from build123d import *

# Parameters (mm, degrees)
ESQUISSE1_R        = 46
BOSS_EXTRU_1_DEPTH = 41
ESQUISSE2_R        = 10
BOSS_EXTRU_2_DEPTH = 1.5
ESQUISSE3_R        = 8
BOSS_EXTRU_3_DEPTH = 3
ESQUISSE4_R        = 0.995
BOSS_EXTRU_4_DEPTH = 3


with BuildPart() as part:
    # Esquisse1 → Boss.-Extru.1 (new body)
    with BuildSketch(Plane(origin=(0, 0, 0), x_dir=(1, 0, 0), z_dir=(0, 1, 0))):
        with Locations(Location((0, 0, 0), (0, 0, 270))):
            Circle(ESQUISSE1_R)
    extrude(amount=BOSS_EXTRU_1_DEPTH)

    # Esquisse2 → Boss.-Extru.2 (add)
    with BuildSketch(Plane(origin=(0, 41, 0), x_dir=(1, 0, 0), z_dir=(0, 1, 0))):
        with Locations(Location((0, 0, 0), (0, 0, 270))):
            Circle(ESQUISSE2_R)
    extrude(amount=BOSS_EXTRU_2_DEPTH)

    # Esquisse3 → Boss.-Extru.3 (add)
    with BuildSketch(Plane(origin=(0, 42.5, 0), x_dir=(1, 0, 0), z_dir=(0, 1, 0))):
        with Locations(Location((0, 0, 0), (0, 0, 270))):
            Circle(ESQUISSE3_R)
    extrude(amount=BOSS_EXTRU_3_DEPTH)

    # Esquisse4 → Boss.-Extru.4 (add)
    with BuildSketch(Plane(origin=(0, 41, 0), x_dir=(1, 0, 0), z_dir=(0, 1, 0))):
        with Locations(Location((0, -31, 0), (0, 0, 270))):
            Circle(ESQUISSE4_R)
    extrude(amount=BOSS_EXTRU_4_DEPTH)


solid = part.part
Can you work these out from the model? Positions are in its coordinate system, mm. A direction names the side the tool comes from. Round coordinates to 2 decimals unless told otherwise and drop trailing zeros. Write each loop counter-clockwise with the first axis right and the second up, starting at its lowest first coordinate (ties: lowest second). Pieces come first, ordered by that corner, then holes. Notation, with made-up numbers: (56, -7) -> (99, -7) arc R31 cw to (99, 17) -> close; hole circle Ø5 at (-21.75, 58.5). An arc over 180 degrees is marked (long way). One line per question, with ' | ' between items. Start each with the question number.
1) Suppose I cut it at C-C on y = 14. Write out the boundary of the cut face in (x, z).
2) Suppose I cut it at A-A on z = 0. Write out the boundary of the cut face in (x, y), then the cut area to 3 significant figures.
3) I need wall thicknesses on line 1 (Y direction, x = -29.5, z = 7.5); line 2 (X direction, y = 38.5, z = 40.5); line 3 (Z direction, x = 9, y = 13). Which ranges of each line are inside material? Lowest first, please. Write a range as [from, to].
4) Suppose I cut it at D-D on z = 34. Write out the boundary of the cut face in (x, y), then the cut area to 3 significant figures.
5) Suppose I cut it at B-B on x = -34.5. Write out the boundary of the cut face in (y, z), then the cut area to 3 significant figures.
6) I'm going to push flat-ended pins straight in: P1, Ø12, axis at y = 26.5, z = -28, coming from the -X side; P2, Ø5, axis at y = 15, z = 32, coming from the +X side; P3, Ø6, axis at x = -3.5, z = -20.5, coming from the +Y side. Where does each tip first touch, or does it pass through?
7) On a 3-axis mill with a long thin cutter (end or side, diameter ignored), from which of +Z, -Z, +X, -X, +Y, -Y can I reach the whole of each face in a straight line? I mean faces 1 (the cylindrical face through (-9.76, 41.74, -2.17)), 2 (the cylindrical face through (38.787, 20.213, 24.729)). Say none if no direction works.
Return value:
1) outline: circle Ø92 at (0, 0)
2) outline: (-46, 0) -> (46, 0) -> (46, 41) -> (10, 41) -> (10, 42.5) -> (8, 42.5) -> (8, 45.5) -> (-8, 45.5) -> (-8, 42.5) -> (-10, 42.5) -> (-10, 41) -> (-46, 41) -> close | area: 3,850 mm2
3) line 1: y = [0, 41] | line 2: x = [-21.81, 21.81] | line 3: z = [-45.11, 45.11]
4) outline: (-30.98, 0) -> (30.98, 0) -> (30.98, 41) -> (-30.98, 41) -> close | area: 2,540 mm2
5) outline: (0, -30.43) -> (41, -30.43) -> (41, 30.43) -> (0, 30.43) -> close | area: 2,490 mm2
6) P1: stops at x = -40.4 | P2: stops at x = 35.3 | P3: stops at y = 41
7) face 1: +Y | face 2: +Y, -Y
